Geometry: final body of the model. Coordinates: model frame, mm. A direction names the side the tool comes from. Give positions to 0.01 mm unless a question says otherwise; leave off trailing zeros. Write each loop counter-clockwise with the first axis right and the second up, starting at its lowest first coordinate (ties: lowest second). Pieces come first, ordered by that corner, then holes. Notation, with made-up numbers: M 43,26.5 L 76,26.5 A26 cw 76,63.5 Z; hole C -9.75,-7.5 d3. An arc over 180 degrees is marked long. Use one line per item in the form item = value. Start each with the question number.
Item 1: Section query B-B on z = -3. Return loops of the section in (x, y), then the cut area to 3 significant figures.
Item 2: Pull-direction query (X, two-part tool) for faces 4 (the flat face through (-25.4, 0, 4)), 5 (the flat face through (0, 0, -3)), 6 (the flat face through (-74, 4.762, 24)); classes: released by +X, released by -X, zero draft, split by the parting line, or undercut.
Item 3: Contact query for flat-ended pins moving along their axis: P1, Ø3, axis at y = 13.5, z = 23.5, coming from the +X side; P2, Ø3, axis at y = -13, z = 14.5, coming from the -X side; P3, Ø4, axis at x = -72.5, z = 26, coming from the -Y side; P4, Ø9, axis at x = -74, y = -0.5, coming from the +Z side. Output: stop coordinate, or through.
Item 4: Section query C-C on x = -46.5. Return loops of the section in (y, z) (1 decimal).
Item 5: Access query for faces 1 (the flat face through (-71, -7.938, 19)), 2 (the flat face through (-6, 0, 10.367)), 3 (the flat face through (-19, 0, -5.08)). Directions: +Z, -Z, +X, -X, +Y, -Y. A direction counts if a zero-diameter tool reaches every point of the face in a straight line with its end or side. Return the directions, or none.
Item 6: Section query D-D on z = 7. Return loops of the section in (x, y).
Item 7: Material intervals for line 1 along X through (y, z) = (6.5, 0.5); line 2 along Y through (x, z) = (-72, 24); line 3 along Z through (x, y) = (-8.5, 10), sorted ascending. Write a range as from..to.
from build123d import *

# Parameters (mm, degrees)
F0_R     = 17.4625
F1_DEPTH = 76.2
F3_DEPTH = 38.1
F5_START = -38.1
F5_DEPTH = 12.7
F7_DEPTH = 25.4


with BuildPart() as f1:
    # F0 (on Right) → F1 (new body)
    with BuildSketch(Plane.YZ):
        Circle(F0_R)
    extrude(amount=-F1_DEPTH)

    # F2 (on Front) → F3 (cut, symmetric)
    with BuildSketch(Plane.XZ):
        Polygon((-12.7, -5.08), (-12.7, 0), (-12.7, 10.3669809178), (0, 10.3669809178), (0, 33.02), (-25.4, 33.02), (-25.4, -5.08), align=None)
    extrude(amount=F3_DEPTH, both=True, mode=Mode.SUBTRACT)

    # F4 (on face) → F5 (join)
    with BuildSketch(Plane.YZ.offset(-25.4).offset(F5_START)):
        with BuildLine():
            Line((-7.9375, 21.9042598667), (-7.9375, 15.5542598667))
            ThreePointArc((-7.9375, 15.5542598667), (9.1194932014, 14.8920700374), (17.4625, 0))
            Line((17.4625, 0), (17.4625, 29.5242598667))
            Line((17.4625, 29.5242598667), (4.7625, 29.5242598667))
            Line((4.7625, 29.5242598667), (4.7625, 21.9042598667))
            Line((4.7625, 21.9042598667), (-7.9375, 21.9042598667))
        make_face()
    extrude(amount=-F5_DEPTH)

    # F6 (on Front) → F7 (cut, symmetric)
    with BuildSketch(Plane.XZ):
        Polygon((-63.5, 29.5242598667), (-76.2, 29.5242598667), (-63.5, 17.4918052011), align=None)
    extrude(amount=F7_DEPTH, both=True, mode=Mode.SUBTRACT)


solid = f1.part
Answer sheet:
q1.outline = M -76.2,-17.2 L -25.4,-17.2 L -25.4,17.2 L -76.2,17.2 Z; M -12.7,-17.2 L 0,-17.2 L 0,17.2 L -12.7,17.2 Z
q1.area = 2,180 mm2
q2.face_4 = undercut
q2.face_5 = released by +X
q2.face_6 = zero draft
q3.P1 = -68.26
q3.P2 = through
q3.P3 = 4.76
q3.P4 = 21.9
q4.outline = C 0,0 d34.9
q5.face_1 = +Z, +X, -X, -Y
q5.face_2 = +Z, +X, +Y, -Y
q5.face_3 = +Z, +Y, -Y
q6.outline = M -76.2,-16 L -25.4,-16 L -25.4,16 L -63.5,16 L -63.5,17.46 L -76.2,17.46 Z; M -12.7,-16 L 0,-16 L 0,16 L -12.7,16 Z
q7.line_1 = -76.2..-25.4, -12.7..0
q7.line_2 = 4.76..17.46
q7.line_3 = -14.32..10.37
